The listing builds one solid part. Answer for the finished solid, in the listing's coordinates (mm). Face numbers are marked on the shaded views. A direction names the side the tool comes from. Give positions to 0.01 mm unless a question says otherwise; leave off trailing zeros. Loops run counter-clockwise (first coordinate to the right, second up) from the corner with the lowest first, then second, coordinate; pieces in that order, holes last. Notation, with made-up numbers: (41, -29) - (73, -29) arc R16 cw to (73, -4) - close; hole circle Ø10 at (74.5, 4). An arc over 180 degrees is marked (long way). Answer as CSV lines item,"result". Start each with the question number.
1) A cutting plane is placed at C-C (x = 49). Determine the outline of the cut face in (y, z).
2) A cutting plane is placed at D-D (y = 59.5). Determine the outline of the cut face in (x, z).
3) For a pull along X with two mould halves and no side action, classify the marked faces 4, 5 and 6 as pulls with the +X half, pulls with the -X half, needs draft (parallel to the pull), parting line crosses it, or undercut.
4) For the marked faces 1, 2 and 3, determine the directions among +Z, -Z, +X, -X, +Y, -Y from which every point of the face is accessible in a straight line to the end or side of a thin tool.
5) Flat-ended cylindrical pins translate along their axes: pin 1 (2 mm diameter, centred on y = 19, z = 20.5, fed in from -X); pin 2 (2.5 mm diameter, centred on x = 113.5, y = 31, fed in from +Z); pin 3 (5 mm diameter, centred on x = 56, y = 31, fed in from +Z). Find the tip coordinate at first contact, or state that the pin passes through.
6) A cutting plane is placed at A-A (y = 69.5). Determine the outline of the cut face in (x, z).
7) A cutting plane is placed at B-B (x = 3). Determine the outline of the cut face in (y, z), and give its area (3 significant figures).
8) Find the intervals of material crossed by line 1 along X through (y, z) = (69.5, 23.85); line 2 along X through (y, z) = (69.5, 21.9); line 3 along Y through (x, z) = (10, 2.5), in increasing order.
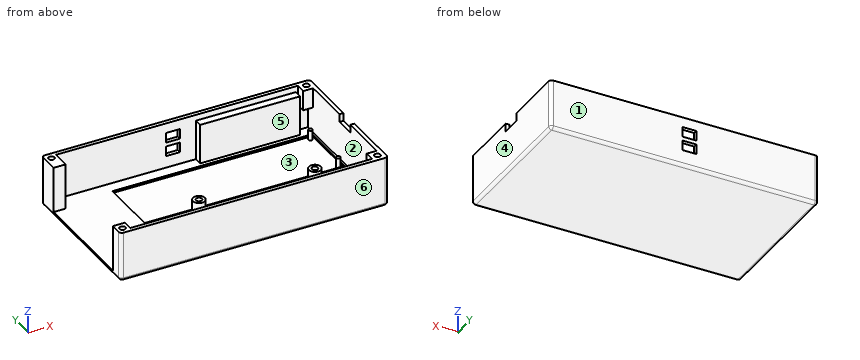
```python
from build123d import *

# Parameters (mm, degrees)
BOX_W             = 134
BOX_H             = 73
BOX_DEPTH         = 25
BOX001_W          = 126
BOX001_H          = 69
BOX001_DEPTH      = 23
BOX002_W          = 10
BOX002_H          = 55
BOX002_DEPTH      = 23
BOX003_W          = 100
BOX003_H          = 30
BOX003_DEPTH      = 1
CYLINDER_R        = 1
CYLINDER_DEPTH    = 5
CYLINDER001_R     = 1
CYLINDER001_DEPTH = 5
CYLINDER002_R     = 3
CYLINDER002_DEPTH = 7
CYLINDER003_R     = 1.5
CYLINDER003_DEPTH = 6
CYLINDER004_R     = 3
CYLINDER004_DEPTH = 7
CYLINDER005_R     = 1.5
CYLINDER005_DEPTH = 6
BOX004_W          = 7
BOX004_H          = 5
BOX004_DEPTH      = 7
BOX005_W          = 7
BOX005_H          = 5
BOX005_DEPTH      = 5
BOX006_W          = 50
BOX006_H          = 20
BOX006_DEPTH      = 4
BOX007_W          = 4
BOX007_H          = 10
BOX007_DEPTH      = 2
CYLINDER006_R     = 1.5
CYLINDER006_DEPTH = 5
CYLINDER007_R     = 1.5
CYLINDER007_DEPTH = 5
BOX008_W          = 5
BOX008_H          = 5
BOX008_DEPTH      = 10
BOX009_W          = 5
BOX009_H          = 5
BOX009_DEPTH      = 10
CYLINDER008_R     = 1.5
CYLINDER008_DEPTH = 5
CYLINDER009_R     = 1.5
CYLINDER009_DEPTH = 5
FILLET_R          = 1.5
FILLET001_R       = 1.5
FILLET002_R       = 1.5
FILLET003_R       = 1.5
CYLINDER010_R     = 6
CYLINDER010_DEPTH = 0.1
CYLINDER011_R     = 6
CYLINDER011_DEPTH = 0.1
BOX010_W          = 12
BOX010_H          = 6
BOX010_DEPTH      = 0.1
CYLINDER012_R     = 5
CYLINDER012_DEPTH = 0.1
CYLINDER013_R     = 8
CYLINDER013_DEPTH = 0.1
CYLINDER014_R     = 5
CYLINDER014_DEPTH = 0.1
CYLINDER015_R     = 6
CYLINDER015_DEPTH = 0.1
CYLINDER016_R     = 5
CYLINDER016_DEPTH = 0.1
PRISM_DEPTH       = 0.1


with BuildPart() as part:
    # Box → Box (join)
    with BuildSketch(Plane.XY):
        with Locations((67, 36.5)):
            Rectangle(BOX_W, BOX_H)
    extrude(amount=BOX_DEPTH)

    # Box001 → Box001 (cut)
    with BuildSketch(Plane(origin=(6, 2, 2), x_dir=(1, 0, 0), z_dir=(0, 0, 1))):
        with Locations((63, 34.5)):
            Rectangle(BOX001_W, BOX001_H)
    extrude(amount=BOX001_DEPTH, mode=Mode.SUBTRACT)

    # Box002 → Box002 (cut)
    with BuildSketch(Plane(origin=(-2, 7, 2), x_dir=(1, 0, 0), z_dir=(0, 0, 1))):
        with Locations((5, 27.5)):
            Rectangle(BOX002_W, BOX002_H)
    extrude(amount=BOX002_DEPTH, mode=Mode.SUBTRACT)

    # Box003 → Box003 (cut)
    with BuildSketch(Plane(origin=(31, 35, 1), x_dir=(1, 0, 0), z_dir=(0, 0, 1))):
        with Locations((50, 15)):
            Rectangle(BOX003_W, BOX003_H)
    extrude(amount=BOX003_DEPTH, mode=Mode.SUBTRACT)

    # Cylinder → Cylinder (join)
    with BuildSketch(Plane(origin=(129, 37, 1), x_dir=(1, 0, 0), z_dir=(0, 0, 1))):
        Circle(CYLINDER_R)
    extrude(amount=CYLINDER_DEPTH)

    # Cylinder001 → Cylinder001 (join)
    with BuildSketch(Plane(origin=(129, 63, 1), x_dir=(1, 0, 0), z_dir=(0, 0, 1))):
        Circle(CYLINDER001_R)
    extrude(amount=CYLINDER001_DEPTH)

    # Cylinder002 → Cylinder002 (join)
    with BuildSketch(Plane(origin=(114, 31, 1), x_dir=(1, 0, 0), z_dir=(0, 0, 1))):
        Circle(CYLINDER002_R)
    extrude(amount=CYLINDER002_DEPTH)

    # Cylinder003 → Cylinder003 (cut)
    with BuildSketch(Plane(origin=(114, 31, 3), x_dir=(1, 0, 0), z_dir=(0, 0, 1))):
        Circle(CYLINDER003_R)
    extrude(amount=CYLINDER003_DEPTH, mode=Mode.SUBTRACT)

    # Cylinder004 → Cylinder004 (join)
    with BuildSketch(Plane(origin=(56, 31, 2), x_dir=(1, 0, 0), z_dir=(0, 0, 1))):
        Circle(CYLINDER004_R)
    extrude(amount=CYLINDER004_DEPTH)

    # Cylinder005 → Cylinder005 (cut)
    with BuildSketch(Plane(origin=(56, 31, 3), x_dir=(1, 0, 0), z_dir=(0, 0, 1))):
        Circle(CYLINDER005_R)
    extrude(amount=CYLINDER005_DEPTH, mode=Mode.SUBTRACT)

    # Box004 → Box004 (cut)
    with BuildSketch(Plane(origin=(61, 74, 8), x_dir=(1, 0, 0), z_dir=(0, -1, 0))):
        with Locations((3.5, 2.5)):
            Rectangle(BOX004_W, BOX004_H)
    extrude(amount=BOX004_DEPTH, mode=Mode.SUBTRACT)

    # Box005 → Box005 (cut)
    with BuildSketch(Plane(origin=(61, 74, 15), x_dir=(1, 0, 0), z_dir=(0, -1, 0))):
        with Locations((3.5, 2.5)):
            Rectangle(BOX005_W, BOX005_H)
    extrude(amount=BOX005_DEPTH, mode=Mode.SUBTRACT)

    # Box006 → Box006 (join)
    with BuildSketch(Plane(origin=(76, 71, 2), x_dir=(1, 0, 0), z_dir=(0, -1, 0))):
        with Locations((25, 10)):
            Rectangle(BOX006_W, BOX006_H)
    extrude(amount=BOX006_DEPTH)

    # Box007 → Box007 (cut)
    with BuildSketch(Plane(origin=(134, 41.5, 25), x_dir=(0, 0, -1), z_dir=(-1, 0, 0))):
        with Locations((2, 5)):
            Rectangle(BOX007_W, BOX007_H)
    extrude(amount=BOX007_DEPTH, mode=Mode.SUBTRACT)

    # Cylinder006 → Cylinder006 (cut)
    with BuildSketch(Plane(origin=(3, 3.5, 20), x_dir=(0, 1, 0), z_dir=(0, 0, 1))):
        Circle(CYLINDER006_R)
    extrude(amount=CYLINDER006_DEPTH, mode=Mode.SUBTRACT)

    # Cylinder007 → Cylinder007 (cut)
    with BuildSketch(Plane(origin=(3, 69.5, 20), x_dir=(0, 1, 0), z_dir=(0, 0, 1))):
        Circle(CYLINDER007_R)
    extrude(amount=CYLINDER007_DEPTH, mode=Mode.SUBTRACT)

    # Box008 → Box008 (join)
    with BuildSketch(Plane(origin=(132, 2, 15), x_dir=(0, 1, 0), z_dir=(0, 0, 1))):
        with Locations((2.5, 2.5)):
            Rectangle(BOX008_W, BOX008_H)
    extrude(amount=BOX008_DEPTH)

    # Box009 → Box009 (join)
    with BuildSketch(Plane(origin=(132, 66, 15), x_dir=(0, 1, 0), z_dir=(0, 0, 1))):
        with Locations((2.5, 2.5)):
            Rectangle(BOX009_W, BOX009_H)
    extrude(amount=BOX009_DEPTH)

    # Cylinder008 → Cylinder008 (cut)
    with BuildSketch(Plane(origin=(130.5, 69.5, 20), x_dir=(0, 1, 0), z_dir=(0, 0, 1))):
        Circle(CYLINDER008_R)
    extrude(amount=CYLINDER008_DEPTH, mode=Mode.SUBTRACT)

    # Cylinder009 → Cylinder009 (cut)
    with BuildSketch(Plane(origin=(130.5, 3.5, 20), x_dir=(0, 1, 0), z_dir=(0, 0, 1))):
        Circle(CYLINDER009_R)
    extrude(amount=CYLINDER009_DEPTH, mode=Mode.SUBTRACT)

    # Fillet
    fillet_edges = [part.edges().sort_by_distance(p)[0] for p in [
        (134, 0, 12.5),
    ]]
    fillet(fillet_edges, radius=FILLET_R)

    # Fillet001
    fillet001_edges = [part.edges().sort_by_distance(p)[0] for p in [
        (66.25, 0, 0),
    ]]
    fillet(fillet001_edges, radius=FILLET001_R)

    # Fillet002
    fillet002_edges = [part.edges().sort_by_distance(p)[0] for p in [
        (134, 73, 13.25),
    ]]
    fillet(fillet002_edges, radius=FILLET002_R)

    # Fillet003
    fillet003_edges = [part.edges().sort_by_distance(p)[0] for p in [
        (0, 36.5, 0),
    ]]
    fillet(fillet003_edges, radius=FILLET003_R)

    # Cylinder010 → Cylinder010 (cut)
    with BuildSketch(Plane(origin=(90.5, 13.5, 1.9), x_dir=(0, 1, 0), z_dir=(0, 0, 1))):
        Circle(CYLINDER010_R)
    extrude(amount=CYLINDER010_DEPTH, mode=Mode.SUBTRACT)

    # Cylinder011 → Cylinder011 (cut)
    with BuildSketch(Plane(origin=(85.5, 13.5, 1.9), x_dir=(0, 1, 0), z_dir=(0, 0, 1))):
        Circle(CYLINDER011_R)
    extrude(amount=CYLINDER011_DEPTH, mode=Mode.SUBTRACT)

    # Box010 → Box010 (cut)
    with BuildSketch(Plane(origin=(91, 7.5, 1.9), x_dir=(0, 1, 0), z_dir=(0, 0, 1))):
        with Locations((6, 3)):
            Rectangle(BOX010_W, BOX010_H)
    extrude(amount=BOX010_DEPTH, mode=Mode.SUBTRACT)

    # Cylinder012 → Cylinder012 (cut)
    with BuildSketch(Plane(origin=(86, 23.5, 1.9), x_dir=(0, 1, 0), z_dir=(0, 0, 1))):
        Circle(CYLINDER012_R)
    extrude(amount=CYLINDER012_DEPTH, mode=Mode.SUBTRACT)

    # Cylinder013 → Cylinder013 (cut)
    with BuildSketch(Plane(origin=(90.5, 15.5, 1.9), x_dir=(0, 1, 0), z_dir=(0, 0, 1))):
        Circle(CYLINDER013_R)
    extrude(amount=CYLINDER013_DEPTH, mode=Mode.SUBTRACT)

    # Cylinder014 → Cylinder014 (join)
    with BuildSketch(Plane(origin=(93.5, 19.5, 1.9), x_dir=(0, 1, 0), z_dir=(0, 0, 1))):
        Circle(CYLINDER014_R)
    extrude(amount=CYLINDER014_DEPTH)

    # Cylinder015 → Cylinder015 (cut)
    with BuildSketch(Plane(origin=(89.5, 13.5, 1.9), x_dir=(0, 1, 0), z_dir=(0, 0, 1))):
        Circle(CYLINDER015_R)
    extrude(amount=CYLINDER015_DEPTH, mode=Mode.SUBTRACT)

    # Cylinder016 → Cylinder016 (cut)
    with BuildSketch(Plane(origin=(86, 23.5, 1.9), x_dir=(0, 1, 0), z_dir=(0, 0, 1))):
        Circle(CYLINDER016_R)
    extrude(amount=CYLINDER016_DEPTH, mode=Mode.SUBTRACT)

    # Prism → Prism (cut)
    with BuildSketch(Plane(origin=(80.5, 22.5, 1.9), x_dir=(0.34202, 0.939693, 0), z_dir=(0, 0, 1))):
        Polygon((3, 0), (-1.5, 2.598076), (-1.5, -2.598076), align=None)
    extrude(amount=PRISM_DEPTH, mode=Mode.SUBTRACT)


solid = part.part
```
Ans:
1,outline,"(0, 1.5) arc R1.5 ccw to (1.5, 0) - (71.5, 0) arc R1.5 ccw to (73, 1.5) - (73, 25) - (71, 25) - (71, 2) - (65, 2) - (65, 1) - (35, 1) - (35, 2) - (2, 2) - (2, 25) - (0, 25) - close"
2,outline,"(0, 1.5) arc R1.5 ccw to (1.5, 0) - (132.5, 0) arc R1.5 ccw to (134, 1.5) - (134, 25) - (132, 25) - (132, 2) - (131, 2) - (131, 1) - (31, 1) - (31, 2) - (0, 2) - close"
3,face 4,"pulls with the +X half"
3,face 5,"undercut"
3,face 6,"needs draft"
4,face 1,"+Z, -Z, +X, -X, +Y"
4,face 2,"none"
4,face 3,"+Z"
5,pin 1,"x = 132"
5,pin 2,"z = 8"
5,pin 3,"z = 9"
6,outline,"(0, 1.5) arc R1.5 ccw to (1.5, 0) - (132.5, 0) arc R1.5 ccw to (134, 1.5) - (134, 25) - (132, 25) - (132, 20) - (129, 20) - (129, 25) - (127, 25) - (127, 15) - (132, 15) - (132, 2) - (126, 2) - (126, 22) - (76, 22) - (76, 2) - (6, 2) - (6, 25) - (4.5, 25) - (4.5, 20) - (1.5, 20) - (1.5, 25) - (0, 25) - close"
7,outline,"(0, 1.5) arc R1.5 ccw to (1.5, 0) - (71.5, 0) arc R1.5 ccw to (73, 1.5) - (73, 25) - (71, 25) - (71, 20) - (68, 20) - (68, 25) - (62, 25) - (62, 2) - (7, 2) - (7, 25) - (5, 25) - (5, 20) - (2, 20) - (2, 25) - (0, 25) - close"
7,area,"529 mm2"
8,line 1,"0 to 1.5, 4.5 to 6, 127 to 129, 132 to 134"
8,line 2,"0 to 1.5, 4.5 to 6, 76 to 126, 127 to 129, 132 to 134"
8,line 3,"0 to 2, 71 to 73"
